```python
from build123d import *

# Parameters (mm, degrees)
SKETCH2_W               = 6
SKETCH2_H               = 17
CUT_EXTRUDE1_DEPTH      = 13.475
CUT_EXTRUDE1_DEPTH_BACK = 13.475
SKETCH3_R               = 4
CUT_EXTRUDE2_DEPTH      = 13.475
CUT_EXTRUDE2_DEPTH_BACK = 13.475
CHAMFER1_SIZE           = 0.5


with BuildPart() as part:
    # Sketch1 → Revolve1 (revolve)
    with BuildSketch(Plane.XY, mode=Mode.PRIVATE) as revolve1_sk:
        Polygon((-9.1, 0), (-9.1, -2), (-6.2, -2), (-6.5, 0), (0, 0), (0, -24), (-12.475, -24), (-12.475, -9), (-10.7, -9), (-10.7, 0), align=None)
    revolve(revolve1_sk.sketch.rotate(Axis((0, 0, 0), (0, -1, 0)), 270), axis=Axis((0, 0, 0), (0, -1, 0)))  # turned: the seam where the file's is

    # Sketch2 → Cut-Extrude1 (cut, two sides)
    with BuildSketch(Plane.XY) as cut_extrude1_sk:
        with Locations((0, -15.5)):
            Rectangle(SKETCH2_W, SKETCH2_H)
    extrude(amount=CUT_EXTRUDE1_DEPTH, mode=Mode.SUBTRACT)
    extrude(cut_extrude1_sk.sketch, amount=-CUT_EXTRUDE1_DEPTH_BACK, mode=Mode.SUBTRACT)

    # Sketch3 → Cut-Extrude2 (cut, two sides)
    with BuildSketch(Plane(origin=(0, 0, 0), x_dir=(0, 0, -1), z_dir=(1, 0, 0))) as cut_extrude2_sk:
        with Locations((0, -16)):
            Circle(SKETCH3_R)
    extrude(amount=CUT_EXTRUDE2_DEPTH, mode=Mode.SUBTRACT)
    extrude(cut_extrude2_sk.sketch, amount=-CUT_EXTRUDE2_DEPTH_BACK, mode=Mode.SUBTRACT)

    # Chamfer1
    chamfer1_edges = [part.edges().sort_by_distance(p)[0] for p in [
        (12.475, -24, 0),
        (-12.475, -24, 0),
    ]]
    chamfer(chamfer1_edges, length=CHAMFER1_SIZE)


solid = part.part
```
For this review, take the finished solid that the model builds, in its own axes (mm). A direction names the side the tool comes from. Round coordinates to 2 decimals unless told otherwise and drop trailing zeros. Write each loop counter-clockwise with the first axis right and the second up, starting at its lowest first coordinate (ties: lowest second). Pieces come first, ordered by that corner, then holes.
1) Insertion check: pin 1 Ø5 at (y, z) = (-11.5, -5) entering from +X; pin 2 Ø1.5 at (y, z) = (-8, -5.5) entering from -X; pin 3 Ø6 at (y, z) = (-6.5, 4.5) entering from +X; pin 4 Ø7 at (y, z) = (-16, 0) entering from -X. Each pin has a flat end and moves straight along its axis. Give the tip position at first contact, or say it passes through.
Answer below:
pin 1: stops at x = 12.22
pin 2: stops at x = -9.59
pin 3: stops at x = 12.15
pin 4: passes through
2) Machinability: for faces 1 (the face through (3, -11.8, -0.2)), 2 (the face through (11, -9, 1)), 3 (the face through (5.54, -1.01, -7.22)), 4 (the face through (-11, -9, 0)), which of the approach directions +Z, -Z, +X, -X, +Y, -Y give a long, thin tool a straight path to every point of the face, cutting with its end or side? Answer none if there is none.
Answer below:
face 1: +Z, -Z, -Y
face 2: +X, +Y
face 3: +Y
face 4: -X, +Y
3) Take a section at A-A on z = 0. State how many separate pieces and enclosed holes the cut face has, then the cut area to 3 significant figures.
Answer below:
separate pieces: 3
enclosed holes: 0
area: 302 mm2
4) For line 1 along Y through (x, z) = (-8.25, 0); line 2 along X through (y, z) = (-1.1, 0) (3 decimals); line 3 along Y through (x, z) = (10, 0), list the stretches that pass through material, from the lowest coordinate up.
Answer below:
line 1: y = -24 to -20, -12 to -2
line 2: x = -10.7 to -9.1, -6.335 to 6.335, 9.1 to 10.7
line 3: y = -24 to -20, -12 to 0
5) Take a section at C-C on y = -18.75. Give the boundary of the cut face in (x, z) (3 decimals).
Answer below:
outline: (-12.132, -2.905) arc R12.475 ccw to (-3, -12.109) - (-3, -2.905) - close; (-12.132, 2.905) - (-3, 2.905) - (-3, 12.109) arc R12.475 ccw to start; (3, -12.109) arc R12.475 ccw to (12.132, -2.905) - (3, -2.905) - close; (3, 2.905) - (12.132, 2.905) arc R12.475 ccw to (3, 12.109) - close
6) Take a section at B-B on y = -16. Give the boundary of the cut face in (x, z) (3 decimals), then the cut area to 3 significant figures.
Answer below:
outline: (-11.816, -4) arc R12.475 ccw to (-3, -12.109) - (-3, -4) - close; (-11.816, 4) - (-3, 4) - (-3, 12.109) arc R12.475 ccw to start; (3, -12.109) arc R12.475 ccw to (11.816, -4) - (3, -4) - close; (3, 4) - (11.816, 4) arc R12.475 ccw to (3, 12.109) - close
area: 193 mm2
7) Take a section at D-D on y = -2.5. Give the boundary of the cut face in (x, z), then the cut area to 3 significant figures.
Answer below:
outline: circle Ø21.4 at (0, 0)
area: 360 mm2
8) Mouldability with a two-part tool opening along Z and no side actions: class faces 5 (the face through (0, 0, 0)), 6 (the face through (4.098, -4.437, 9.884)), 7 (the face through (4, -2, 6)) as +Z half, -Z half, draft (parallel to the pull), parting line (faces both ways), or undercut.
Answer below:
face 5: draft
face 6: parting line
face 7: undercut
